Check sheet for the drawn part. Datum: minimum x, y, z corner. Units: mm. A direction names the side the tool comes from. Give positions to 0.01 mm unless a question says otherwise; leave off trailing zeros. Write each loop counter-clockwise with the first axis right and the second up, starting at its lowest first coordinate (ties: lowest second). Pieces come first, ordered by that corner, then holes.
(1) Cross-section at D-D (x = 42.5). Record the boundary of the cut face in (y, z) (1 decimal), and give its area (3 significant figures).
(2) Cross-section at C-C (y = 4). Record the boundary of the cut face in (x, z).
(3) Thickness scan on line 1 along Y through (x, z) = (43, 28); line 2 along Y through (x, z) = (19, 40.5); line 3 along X through (y, z) = (9.5, 22) (1 decimal). Record the ranges inside material, lowest first.
(4) Depth check by flat-ended pin: P1, Ø10, axis at y = 7.5, z = 40, coming from the -X side; P2, Ø3, axis at y = 6, z = 14, coming from the +X side; P3, Ø5.5, axis at x = 52.84, z = 25.84, coming from the -Y side; P4, Ø12, axis at x = 45.5, z = 42.5, coming from the -Y side. Enter the tip coordinate at first touch or a pass-through.
(5) Tool access check on the marked faces 1 and 2. Record the directions out of +Z, -Z, +X, -X, +Y, -Y that give a thin tool (end or side, any length) a straight path to the whole face; none if there is none.
(6) Cross-section at A-A (x = 59). Record the boundary of the cut face in (y, z) (1 decimal).
(7) Cross-section at B-B (z = 35). Record the boundary of the cut face in (x, y) (1 decimal).
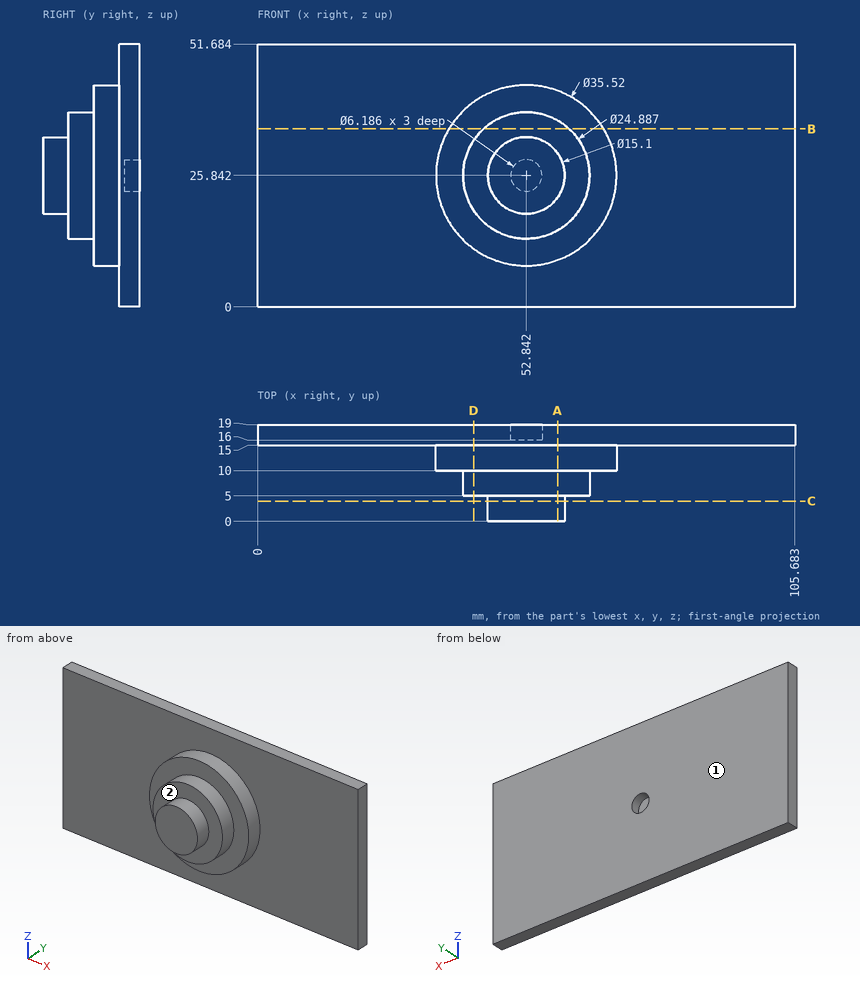
Reply:
1. outline: (5, 18.9) - (10, 18.9) - (10, 11.4) - (15, 11.4) - (15, 0) - (19, 0) - (19, 51.7) - (15, 51.7) - (15, 40.3) - (10, 40.3) - (10, 32.8) - (5, 32.8) - close
1. area: 420 mm2
2. outline: circle Ø15.1 at (52.84, 25.84)
3. line 1: y = 5 to 19
3. line 2: y = 15 to 19
3. line 3: x = 41 to 64.7
4. P1: stops at x = 38.05
4. P2: stops at x = 59.76
4. P3: stops at y = 0
4. P4: stops at y = 5
5. face 1: +Z, -Z, +X, -X, +Y
5. face 2: -Y
6. outline: (0, 21.5) - (5, 21.5) - (5, 15) - (10, 15) - (10, 9.2) - (15, 9.2) - (15, 0) - (19, 0) - (19, 51.7) - (15, 51.7) - (15, 42.5) - (10, 42.5) - (10, 36.7) - (5, 36.7) - (5, 30.2) - (0, 30.2) - close
7. outline: (0, 15) - (37.6, 15) - (37.6, 10) - (44.4, 10) - (44.4, 5) - (61.3, 5) - (61.3, 10) - (68.1, 10) - (68.1, 15) - (105.7, 15) - (105.7, 19) - (0, 19) - close
